Source: CAD feature listing. Evaluate the final solid. Frame: model axes, mm. A direction names the side the tool comes from. Give positions to 0.01 mm unless a question says otherwise; leave off trailing zeros. Order: outer loops, then holes, each group sorted by start corner. A loop starts at its lowest first (then second) coordinate and runs counter-clockwise, first axis right, second up. Notation, with made-up numbers: (11, 1) -> (47, 1) arc R24 ccw to (47, 31) -> close; hole circle Ø9 at (6.25, 44.5). An arc over 180 degrees is marked (long way). Answer in a Markdown table with one row per item.
```python
from build123d import *

# Parameters (mm, degrees)
EXTRUDE_1_DEPTH          = 60
CUT_EXTRUDE_1_DEPTH      = 40
CUT_EXTRUDE_1_DEPTH_BACK = 29
SKETCH_4_R               = 15.5
SKETCH_5_W               = 5
SKETCH_5_H               = 30
CUT_EXTRUDE_2_DEPTH      = 83.900874001
SKETCH_7_W               = 60
SKETCH_7_H               = 85.424918669
EXTRUDE_2_DEPTH          = 17
CUT_EXTRUDE_START        = -34.454396
SKETCH_9_W               = 21
SKETCH_9_H               = 39
CUT_EXTRUDE_3_DEPTH      = 14
CUT_EXTRUDE_START_2      = -15
SKETCH_14_W              = 60
SKETCH_14_H              = 56
CUT_EXTRUDE_8_DEPTH      = 10
CUT_EXTRUDE_START_3      = 15
SKETCH_16_W              = 60
SKETCH_16_H              = 39
CUT_EXTRUDE_11_DEPTH     = 10
EXTRUDE_START            = -34.454396
EXTRUDE_5_DEPTH          = 6


with BuildPart() as part:
    # 스케치3 → 보스-돌출1 (new body)
    with BuildSketch(Plane(origin=(0, 0, 0), x_dir=(0, 0, -1), z_dir=(1, 0, 0))):
        Polygon((-25, -51.454396413), (25, -51.454396413), (15, 4.545603587), (-15, 4.545603587), align=None)
    extrude(amount=EXTRUDE_1_DEPTH)

    # 스케치4 → 컷-돌출1 (cut, two sides: drawn at the far end of the back side and taken through both)
    with BuildSketch(Plane.XY.offset(-CUT_EXTRUDE_1_DEPTH_BACK)):
        with Locations(Location((30, -14.954396413, 0), (0, 0, 90))):
            Circle(SKETCH_4_R)
    extrude(amount=CUT_EXTRUDE_1_DEPTH + CUT_EXTRUDE_1_DEPTH_BACK, mode=Mode.SUBTRACT)

    # 스케치5 → 컷-돌출2 (cut, through all)
    with BuildSketch(Plane(origin=(0, 0, 0), x_dir=(0, 0, -1), z_dir=(1, 0, 0))):
        with Locations((0, -51.454396413)):
            Rectangle(SKETCH_5_W, SKETCH_5_H)
    extrude(amount=CUT_EXTRUDE_2_DEPTH, mode=Mode.SUBTRACT)

    # 스케치7 → 보스-돌출2 (add)
    with BuildSketch(Plane(origin=(0, -51.454396413, 0), x_dir=(-1, 0, 0), z_dir=(0, -1, 0))):
        with Locations((-30, -47.287540666)):
            Rectangle(SKETCH_7_W, SKETCH_7_H)
    extrude(amount=-EXTRUDE_2_DEPTH)

    # 스케치9 → 컷-돌출3 (cut)
    with BuildSketch(Plane(origin=(0, 0, 0), x_dir=(1, 0, 0), z_dir=(0, 1, 0)).offset(CUT_EXTRUDE_START)):
        with Locations((30, -55.464285714)):
            Rectangle(SKETCH_9_W, SKETCH_9_H)
    extrude(amount=-CUT_EXTRUDE_3_DEPTH, mode=Mode.SUBTRACT)

    # 스케치14 → 컷-돌출8 (cut)
    with BuildSketch(Plane.XY.offset(CUT_EXTRUDE_START_2)):
        with Locations((30, -23.454396413)):
            Rectangle(SKETCH_14_W, SKETCH_14_H)
    extrude(amount=-CUT_EXTRUDE_8_DEPTH, mode=Mode.SUBTRACT)

    # 스케치16 → 컷-돌출11 (cut)
    with BuildSketch(Plane.XY.offset(CUT_EXTRUDE_START_3)):
        with Locations((30, -14.954396413)):
            Rectangle(SKETCH_16_W, SKETCH_16_H)
    extrude(amount=CUT_EXTRUDE_11_DEPTH, mode=Mode.SUBTRACT)


with BuildPart() as extrude_5_tool:
    # 스케치17 → 보스-돌출5 (new body)
    with BuildSketch(Plane(origin=(0, 0, 0), x_dir=(1, 0, 0), z_dir=(0, 1, 0)).offset(EXTRUDE_START)):
        Polygon((19.5, -35.964285714), (0, -35.964285714), (0, -90), (60, -90), (60, -35.964285714), (40.5, -35.964285714), (40.5, -74.964285714), (19.5, -74.964285714), align=None)
    extrude(amount=EXTRUDE_5_DEPTH)


with BuildPart() as part_1:
    add(part.part)


with BuildPart() as part_2:
    # 보스-돌출5: joined with extrude_5_tool
    add(part_1.part.fuse(extrude_5_tool.part, tol=0.00001))


solid = part_2.part
```
(1) Pull-direction query (Z, two-part tool) for faces 5 (the flat face through (23, -29, -15)), 6 (the flat face through (30, -40, 90)), 7 (the flat face through (30, -51.454, -9)), 8 (the flat face through (10, -31, 35.964)); classes: +Z half, -Z half, draft (parallel to the pull), parting line (faces both ways), or undercut.
A:
| item | result |
|---|---|
| face 5 | -Z half |
| face 6 | +Z half |
| face 7 | draft |
| face 8 | undercut |
(2) First-contact query: pin 1 Ø19.5 at (x, y) = (21.5, -8.5) entering from +Z; pin 2 Ø2 at (x, z) = (14, 25) entering from +Y; pin 3 Ø10 at (y, z) = (-26.5, 37.5) entering from +X; pin 4 Ø2.5 at (x, z) = (42, -0.5) entering from -Y. Flat tips, straight axial feed; report the tip coordinate or a pass-through.
A:
| item | result |
|---|---|
| pin 1 | stops at z = 15 |
| pin 2 | stops at y = -34.45 |
| pin 3 | stops at x = 60 |
| pin 4 | stops at y = -36.45 |
(3) Section query A-A (x = 30). Return the cut outline in (y, z), plus the area to 3 significant figures.
A:
| item | result |
|---|---|
| outline | (-51.45, -15) -> (-30.45, -15) -> (-30.45, 15) -> (-34.45, 15) -> (-34.45, 35.96) -> (-48.45, 35.96) -> (-48.45, 74.96) -> (-28.45, 74.96) -> (-28.45, 90) -> (-51.45, 90) -> (-51.45, 2.5) -> (-36.45, 2.5) -> (-36.45, -2.5) -> (-51.45, -2.5) -> close; (0.55, -15) -> (4.55, -15) -> (4.55, 15) -> (0.55, 15) -> close |
| area | 1,490 mm^2 |
(4) Section query C-C (z = 46.5). Return the cut outline in (x, y), plus the area to 3 significant figures.
A:
| item | result |
|---|---|
| outline | (0, -51.45) -> (60, -51.45) -> (60, -28.45) -> (40.5, -28.45) -> (40.5, -48.45) -> (19.5, -48.45) -> (19.5, -28.45) -> (0, -28.45) -> close |
| area | 960 mm^2 |
(5) Section query D-D (y = -3.5). Return the cut outline in (x, z), plus the area to 3 significant figures.
A:
| item | result |
|---|---|
| outline | (0, -15) -> (19.56, -15) -> (19.56, 15) -> (0, 15) -> close; (40.44, -15) -> (60, -15) -> (60, 15) -> (40.44, 15) -> close |
| area | 1,170 mm^2 |
(6) Access query for faces 1 (the flat face through (30, 4.546, 0)), 2 (the flat face through (30, -39, 74.964)), 3 (the flat face through (30, -36.454, 0)), 4 (the flat face through (16, -6, 15)). Directions: +Z, -Z, +X, -X, +Y, -Y. A direction counts if a zero-diameter tool reaches every point of the face in a straight line with its end or side. Return the directions, or none.
A:
| item | result |
|---|---|
| face 1 | +Z, -Z, +X, -X, +Y |
| face 2 | +Y |
| face 3 | +X, -X, -Y |
| face 4 | +X, -X, +Y |
(7) Section query B-B (y = -39). Return the cut outline in (x, z), plus the area to 3 significant figures.
A:
| item | result |
|---|---|
| outline | (0, -15) -> (60, -15) -> (60, -2.5) -> (0, -2.5) -> close; (0, 2.5) -> (60, 2.5) -> (60, 90) -> (0, 90) -> close; hole (19.5, 35.96) -> (40.5, 35.96) -> (40.5, 74.96) -> (19.5, 74.96) -> close |
| area | 5,180 mm^2 |
(8) Ray query, probe 1 along X at (y, z) = (-42.5, 36); probe 2 along Z at (x, y) = (55, -37); probe 3 along Z at (x, y) = (45, -32.5). Return the intervals inside material, ascending.
A:
| item | result |
|---|---|
| probe 1 | x = 0 to 19.5, 40.5 to 60 |
| probe 2 | z = -15 to -2.5, 2.5 to 90 |
| probe 3 | z = -15 to 15, 35.96 to 90 |
